```python
from build123d import *

# Parameters (mm, degrees)
ESQUISSE1_W        = 5
ESQUISSE1_H        = 3
BOSS_EXTRU_1_DEPTH = 3


with BuildPart() as part:
    # Esquisse1 → Boss.-Extru.1 (new body)
    with BuildSketch(Plane.XY):
        Polygon((-127.914818772, 46.520106884), (-127.914818772, 36.520106884), (-132.914818772, 36.520106884), (-132.914818772, 46.520106884), (-137.914818772, 46.520106884), (-137.914818772, 19.020106884), (-22.914818772, 19.020106884), (-22.914818772, 46.520106884), (-27.914818772, 46.520106884), (-27.914818772, 36.520106884), (-32.914818772, 36.520106884), (-32.914818772, 46.520106884), (-37.914818772, 46.520106884), (-37.914818772, 36.520106884), (-42.914818772, 36.520106884), (-42.914818772, 46.520106884), (-47.914818772, 46.520106884), (-47.914818772, 36.520106884), (-52.914818772, 36.520106884), (-52.914818772, 46.520106884), (-57.914818772, 46.520106884), (-57.914818772, 36.520106884), (-62.914818772, 36.520106884), (-62.914818772, 46.520106884), (-67.914818772, 46.520106884), (-67.914818772, 36.520106884), (-72.914818772, 36.520106884), (-72.914818772, 46.520106884), (-77.914818772, 46.520106884), (-77.914818772, 36.520106884), (-82.914818772, 36.520106884), (-82.914818772, 46.520106884), (-87.914818772, 46.520106884), (-87.914818772, 36.520106884), (-92.914818772, 36.520106884), (-92.914818772, 46.520106884), (-97.914818772, 46.520106884), (-97.914818772, 36.520106884), (-102.914818772, 36.520106884), (-102.914818772, 46.520106884), (-107.914818772, 46.520106884), (-107.914818772, 36.520106884), (-112.914818772, 36.520106884), (-112.914818772, 46.520106884), (-117.914818772, 46.520106884), (-117.914818772, 36.520106884), (-122.914818772, 36.520106884), (-122.914818772, 46.520106884), align=None)
        with Locations((-30.414818772, 30.020106884)):
            Rectangle(ESQUISSE1_W, ESQUISSE1_H, mode=Mode.SUBTRACT)
        with Locations((-40.414818772, 30.020106884)):
            Rectangle(ESQUISSE1_W, ESQUISSE1_H, mode=Mode.SUBTRACT)
        with Locations((-50.414818772, 30.020106884)):
            Rectangle(ESQUISSE1_W, ESQUISSE1_H, mode=Mode.SUBTRACT)
        with Locations((-60.414818772, 30.020106884)):
            Rectangle(ESQUISSE1_W, ESQUISSE1_H, mode=Mode.SUBTRACT)
        with Locations((-70.414818772, 30.020106884)):
            Rectangle(ESQUISSE1_W, ESQUISSE1_H, mode=Mode.SUBTRACT)
        with Locations((-80.414818772, 30.020106884)):
            Rectangle(ESQUISSE1_W, ESQUISSE1_H, mode=Mode.SUBTRACT)
        with Locations((-90.414818772, 30.020106884)):
            Rectangle(ESQUISSE1_W, ESQUISSE1_H, mode=Mode.SUBTRACT)
        with Locations((-100.414818772, 30.020106884)):
            Rectangle(ESQUISSE1_W, ESQUISSE1_H, mode=Mode.SUBTRACT)
        with Locations((-30.414818772, 25.520106884)):
            Rectangle(ESQUISSE1_W, ESQUISSE1_H, mode=Mode.SUBTRACT)
        with Locations((-40.414818772, 25.520106884)):
            Rectangle(ESQUISSE1_W, ESQUISSE1_H, mode=Mode.SUBTRACT)
        with Locations((-50.414818772, 25.520106884)):
            Rectangle(ESQUISSE1_W, ESQUISSE1_H, mode=Mode.SUBTRACT)
        with Locations((-60.414818772, 25.520106884)):
            Rectangle(ESQUISSE1_W, ESQUISSE1_H, mode=Mode.SUBTRACT)
        with Locations((-70.414818772, 25.520106884)):
            Rectangle(ESQUISSE1_W, ESQUISSE1_H, mode=Mode.SUBTRACT)
        with Locations((-80.414818772, 25.520106884)):
            Rectangle(ESQUISSE1_W, ESQUISSE1_H, mode=Mode.SUBTRACT)
        with Locations((-90.414818772, 25.520106884)):
            Rectangle(ESQUISSE1_W, ESQUISSE1_H, mode=Mode.SUBTRACT)
        with Locations((-100.414818772, 25.520106884)):
            Rectangle(ESQUISSE1_W, ESQUISSE1_H, mode=Mode.SUBTRACT)
        with Locations((-110.414818772, 25.520106884)):
            Rectangle(ESQUISSE1_W, ESQUISSE1_H, mode=Mode.SUBTRACT)
        with Locations((-120.414818772, 25.520106884)):
            Rectangle(ESQUISSE1_W, ESQUISSE1_H, mode=Mode.SUBTRACT)
        with Locations((-110.414818772, 30.020106884)):
            Rectangle(ESQUISSE1_W, ESQUISSE1_H, mode=Mode.SUBTRACT)
        with Locations((-130.414818772, 25.520106884)):
            Rectangle(ESQUISSE1_W, ESQUISSE1_H, mode=Mode.SUBTRACT)
        with Locations((-120.414818772, 30.020106884)):
            Rectangle(ESQUISSE1_W, ESQUISSE1_H, mode=Mode.SUBTRACT)
        with Locations((-130.414818772, 30.020106884)):
            Rectangle(ESQUISSE1_W, ESQUISSE1_H, mode=Mode.SUBTRACT)
    extrude(amount=BOSS_EXTRU_1_DEPTH)


solid = part.part
```
Can you work these out from the model? Positions are in its coordinate system, mm. A direction names the side the tool comes from. Coordinates: 2 decimals unless noted, no trailing zeros. Order: outer loops, then holes, each group sorted by start corner. A loop starts at its lowest first (then second) coordinate and runs counter-clockwise, first axis right, second up.
1. I need wall thicknesses on line 1 (Y direction, x = -62.5, z = 2.1). Which ranges of the line are inside material? Lowest first, please.
2. For faces 3 (the face through (-92.915, 41, 1)), 4 (the face through (-42.915, 25, 1)), which set-ups out of +Z, -Z, +X, -X, +Y, -Y let a thin tool reach every point of the face, with its end or its side?
3. Thinking about a two-plate mould opening in X: for faces 1 (the face through (-57.915, 42, 1)), 2 (the face through (-81, 33, 3)), which applies, +X half, -X half, draft (parallel to the pull), parting line (faces both ways), or undercut?
4. If we section it at A-A (x = -91.5): Please give me the cut outline in (y, z), then the cut area to 3 significant figures.
5. If we section it at B-B (y = 30.5): Give the number of separate pieces and of enclosed holes in the cut face, then the cut area to 3 significant figures.
6. I'm going to push flat-ended pins straight in: pin 1 (0.9 mm diameter, centred on x = -50, z = 2, fed in from +Y); pin 2 (1 mm diameter, centred on x = -92, y = 39, fed in from -Z). Where does each tip first touch, or does it pass through?
Entries:
1. line 1: y = 19.02 to 24.02, 27.02 to 28.52, 31.52 to 36.52
2. face 3: +Z, -Z, +Y
2. face 4: +Z, -Z
3. face 1: undercut
3. face 2: draft
4. outline: (19.02, 0) - (24.02, 0) - (24.02, 3) - (19.02, 3) - close; (27.02, 0) - (28.52, 0) - (28.52, 3) - (27.02, 3) - close; (31.52, 0) - (36.52, 0) - (36.52, 3) - (31.52, 3) - close
4. area: 34.5 mm2
5. separate pieces: 12
5. enclosed holes: 0
5. area: 180 mm2
6. pin 1: stops at y = 36.52
6. pin 2: passes through
